For this review, use the dimensioned drawing (mm, ordinates from the lowest corner) and the shaded views. A direction names the side the tool comes from. Coordinates: 2 decimals unless noted, no trailing zeros. Order: outer loops, then holes, each group sorted by start corner. A loop starts at its lowest first (then second) coordinate and runs counter-clockwise, first axis right, second up. Notation, with made-up numbers: M -34,37 L -17,37 A20 cw -17,69 Z; hole C 67.25,29.25 d3. An arc over 180 degrees is marked long. Write each question's results on one line, items separated by ' | '.
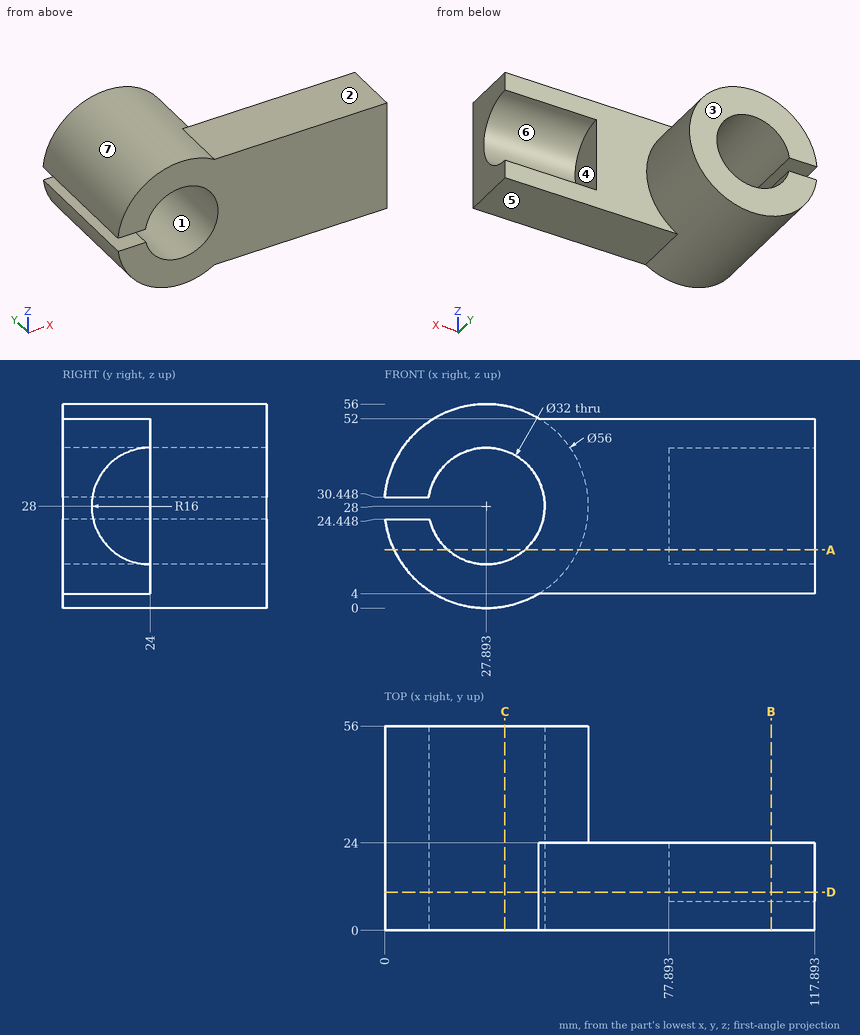
1) Take a section at A-A on z = 16. State the section outline as (x, y) points (1 decimal).
Solutions:
outline: M 2.6,0 L 17.3,0 L 17.3,56 L 2.6,56 Z; M 38.5,0 L 117.9,0 L 117.9,13.4 L 77.9,13.4 L 77.9,24 L 53.2,24 L 53.2,56 L 38.5,56 Z
2) To check wall thickness, follow line 1 along Z through (x, y) = (87, 23.5); line 2 along Z through (x, y) = (64.5, 3); line 3 along X through (y, z) = (34, 28). State the ranges of each line that lie inside material, in increasing order.
Solutions:
line 1: 4 to 12.01, 43.99 to 52 | line 2: 4 to 52 | line 3: 43.89 to 55.89
3) Take a section at B-B on x = 106. State the section outline as (y, z) points, plus the area to 3 significant figures.
Solutions:
outline: M 0,4 L 24,4 L 24,12 A16 cw 24,44 L 24,52 L 0,52 Z | area: 750 mm2
4) The part is to be moulded in two halves that separate along Z. For the marked faces 1, 2, 3 and 4, say which applies: pulls with the +Z half, pulls with the -Z half, needs draft (parallel to the pull), parting line crosses it, or undercut.
Solutions:
face 1: undercut | face 2: pulls with the +Z half | face 3: needs draft | face 4: undercut
5) For the marked faces 5, 6 and 7, list the 3-axis set-ups (+Z, -Z, +X, -X, +Y, -Y) from which the entire face can be reached by the end or side of a thin tool; tool diameter is ignored.
Solutions:
face 5: -Z, +X, +Y, -Y | face 6: +X, +Y | face 7: +Y
6) Take a section at C-C on x = 33. State the section outline as (y, z) points, plus the area to 3 significant figures.
Solutions:
outline: M 0,0.47 L 56,0.47 L 56,12.84 L 0,12.84 Z; M 0,43.16 L 56,43.16 L 56,55.53 L 0,55.53 Z | area: 1,390 mm2
7) Take a section at D-D on y = 10.5. State the section outline as (x, z) points (1 decimal), plus the area to 3 significant figures.
Solutions:
outline: M 0,30.4 L 12.1,30.4 A16 cw long 12.3,24.4 L 0.1,24.4 A28 ccw 42.3,4 L 117.9,4 L 117.9,19.4 L 77.9,19.4 L 77.9,36.6 L 117.9,36.6 L 117.9,52 L 42.3,52 A28 ccw Z | area: 4,070 mm2
8) For pin 1 (2 mm diameter, centred on x = 83.5, z = 10, fed in from +Y); pin 2 (1 mm diameter, centred on y = 46.5, z = 44, fed in from -X) (1 decimal); pin 3 (13.5 mm diameter, centred on x = 5, y = 27, fed in from +Z), all flat-tipped, find the tip position at first contact; note any pin that passes through.
Solutions:
pin 1: y = 24 | pin 2: x = 4.6 | pin 3: z = 50.88
